Could you check a few things on this drawing? It's one solid part, dimensions in mm from its lowest x, y, z. Give positions to 0.01 mm unless a question says otherwise; leave off trailing zeros. Order: outer loops, then holes, each group sorted by start corner. A loop starts at its lowest first (then second) coordinate and runs counter-clockwise, first axis right, second up. Notation, with made-up numbers: (34, 71) -> (65, 71) arc R12 cw to (65, 94) -> close; hole circle Ø3 at (3.25, 65). An arc over 180 degrees is marked (long way). Answer as a JSON object with one key per item and string values.
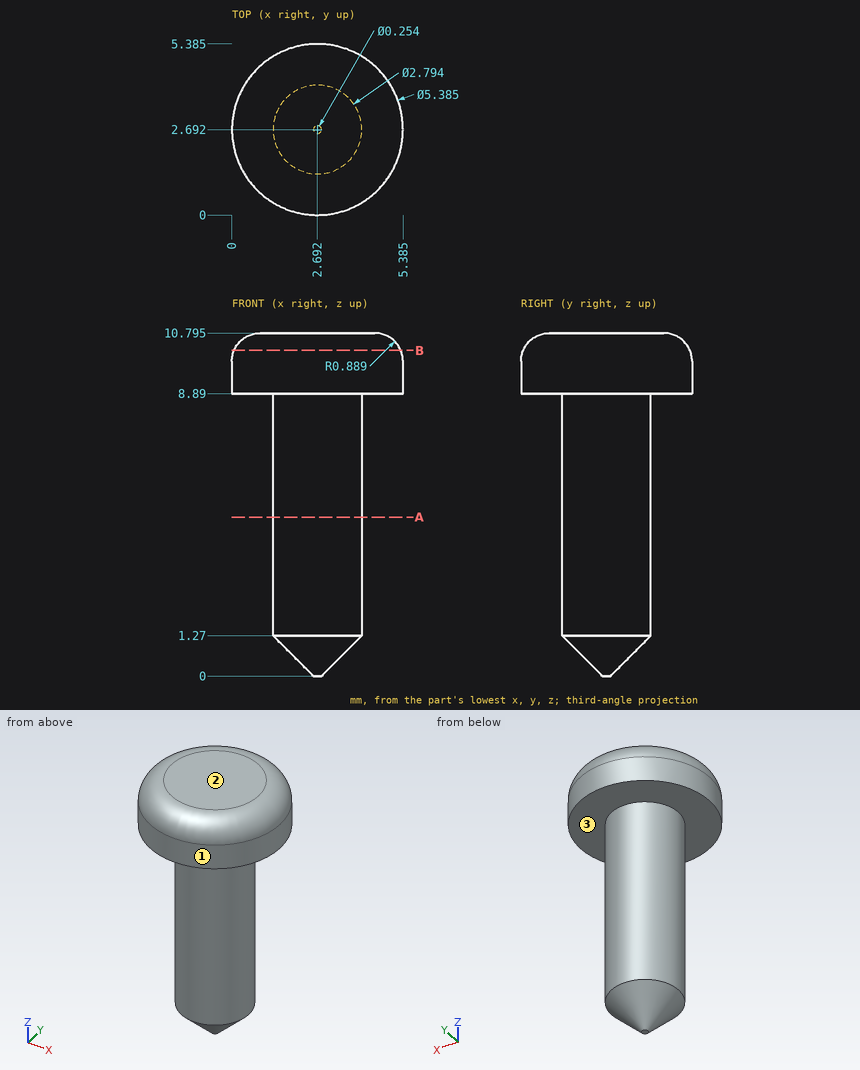
1. Please list where these lines run through material, in increasing order: L1, parallel to Z at x = 1.05, y = 3.45 (1 decimal); L2, parallel to Y at x = 1.25, z = 10.5 (1 decimal); L3, parallel to X at y = 1.5, z = 5.5 (1 decimal).
Worked answers:
{"L1": "8.9 to 10.8", "L2": "0.7 to 4.7", "L3": "2 to 3.4"}
2. If we mould it in two halves opening along Z, with no side actions, what happens to the marked faces 1, 2 and 3? For each: +Z half, -Z half, draft (parallel to the pull), parting line (faces both ways), or undercut.
Worked answers:
{"face 1": "draft", "face 2": "+Z half", "face 3": "-Z half"}
3. If we section it at A-A on z = 5: Please give me the cut outline in (x, y).
Worked answers:
{"outline": "circle Ø2.79 at (2.69, 2.69)"}
4. Will this pin go through, and if not, where does the flat tip stop? pin 1 Ø2 at (y, z) = (3.5, 7) entering from -X (1 decimal).
Worked answers:
{"pin 1": "x = 1.3"}
5. If we section it at B-B on z = 10.25: Please give me the cut outline in (x, y) (1 decimal).
Worked answers:
{"outline": "circle Ø5.2 at (2.7, 2.7)"}
